Can you work these out from the model? Positions are in its coordinate system, mm. Face numbers are marked on the shaded views. A direction names the side the tool comes from. Give positions to 0.01 mm unless a question says otherwise; leave off trailing zeros. Loops run counter-clockwise (first coordinate to the right, second up) from the corner with the lowest first, then second, coordinate; pieces in that order, holes last. Notation, with made-up numbers: (2, 60.5) - (25, 60.5) arc R18 cw to (25, 84.5) - close; hole circle Ø9 at (17.5, -33.5). An arc over 180 degrees is marked (long way). Use a Markdown table: item, result. Add a question column.
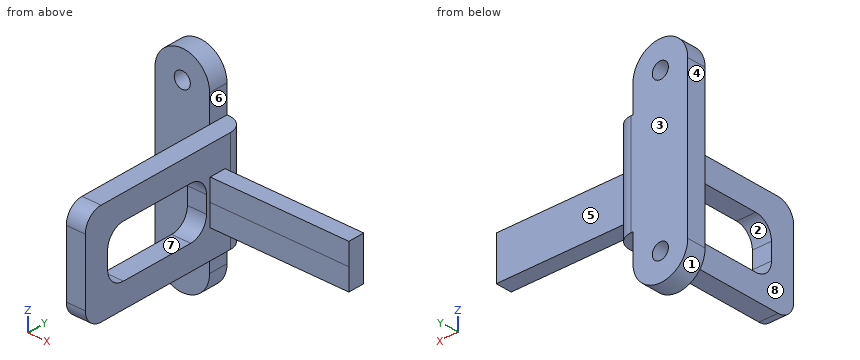
Autodesk Inventor part; units mm, degrees
ref_plane "YZ Plane" through (0, 0, 0) normal (1, 0, 0) x (0, 1, 0)
ref_plane "XZ Plane" through (0, 0, 0) normal (0, 1, 0) x (-1, 0, 0)
ref_plane "XY Plane" through (0, 0, 0) normal (0, 0, 1) x (1, 0, 0)
sketch "Sketch1" plane through (0, 0, 0) normal (0, 1, 0) x (-1, 0, 0)
  circle A0 centre (0, 0) radius 1.4732
  circle A1 centre (0, -28.4988) radius 1.4732
  circle A2 centre (0, 0) radius 5.0165
  circle A3 centre (0, -28.4988) radius 5.0165
  line L0 (5.0165, 0) -> (5.0165, -28.4988)
  line L1 (-5.0165, 0) -> (-5.0165, -28.4988)
  dimension "d0" = 2.9464
  dimension "d2" = 2.9464
  dimension "d3" = 10.033
  dimension "d4" = 10.033
extrude "Extrusion1" add sketch "Sketch1" along normal blind 3.5
sketch "Sketch2" plane through (5.0165, 0, 0) normal (1, 0, 0) x (0, 0, -1)
  line L0 (0, 0) -> (28.4988, 0)
  line L1 (0, 0) -> (5.0292, 0)
  line L2 (28.4988, 0) -> (28.4988, 3.5)
  line L3 (28.4988, 0) -> (23.4696, 0)
  line L4 (23.4696, 0) -> (5.0292, 0)
  line L5 (5.0292, 0) -> (5.0292, -25.7302)
  line L6 (8.2042, -28.9052) -> (20.2946, -28.9052)
  line L7 (23.4696, -25.7302) -> (23.4696, 0)
  line L8 (5.0292, 0) -> (23.4696, 0)
  line L9 (5.0292, 0) -> (11.3792, 0)
  line L10 (23.4696, 0) -> (17.1196, 0)
  line L11 (5.0292, -28.9052) -> (11.3792, -28.9052)
  arc A0 (5.0292, -25.7302) -> (8.2042, -28.9052) centre (8.2042, -25.7302) ccw
  arc A1 (20.2946, -28.9052) -> (23.4696, -25.7302) centre (20.2946, -25.7302) ccw
  line L12 (15.8041, -24.4147) -> (12.694, -24.4147)
  line L13 (12.694, -4.4898) -> (15.8041, -4.4898)
  line L14 (18.9791, -7.6648) -> (18.9791, -21.2397)
  line L15 (9.519, -21.2397) -> (9.519, -7.6648)
  arc A2 (12.694, -4.4898) -> (9.519, -7.6648) centre (12.694, -7.6648) ccw
  arc A3 (9.519, -21.2397) -> (12.694, -24.4147) centre (12.694, -21.2397) ccw
  arc A4 (15.8041, -24.4147) -> (18.9791, -21.2397) centre (15.8041, -21.2397) ccw
  arc A5 (18.9791, -7.6648) -> (15.8041, -4.4898) centre (15.8041, -7.6648) ccw
  point P0 (9.519, -24.4147)
  dimension "d7" = 5.0292
  dimension "d8" = 5.0292
  dimension "d9" = 28.9052
  dimension "d10" = 6.35
  dimension "d14" = 6.35
  dimension "d17" = 3.175
  dimension "d23" = 6.35
  dimension "d25" = 3.175
extrude "Extrusion4" add sketch "Sketch2" along normal blind 3.5
sketch "Sketch4" plane through (5.0165, 0, -5.0292) normal (0, 1, 0) x (1, 0, 0)
  line L0 (0, 0) -> (3.5, 0)
  line L1 (3.5, 15.2654) -> (3.5, 18.4404)
  line L2 (3.5, 0) -> (3.5, 18.4404)
  line L3 (0, 18.4404) -> (3.5, 18.4404)
  line L4 (3.5, 18.4404) -> (0, 18.4404)
  line L5 (0, 18.4404) -> (0, 0)
  line L6 (0, 0) -> (3.5, 0)
  point P0 (-5.0165, -5.0292)
extrude "Extrusion5" add sketch "Sketch4" along normal blind 3.5
fillet "Fillet3" radius 3.175 1 edges at (8.5165, 3.5, -14.2494)
sketch "Sketch5" plane through (8.5165, 0, 0) normal (1, 0, 0) x (0, 0, -1)
  line L0 (5.0292, 0) -> (23.4696, 0)
  line L1 (12.694, -4.4898) -> (15.8041, -4.4898)
  line L2 (14.2491, -3.7449) -> (10.2491, -3.7446)
  line L3 (14.2491, -3.7449) -> (18.2491, -3.7449)
  line L4 (14.2493, -0.7449) -> (10.2491, -0.7449)
  line L5 (10.2491, -0.7449) -> (10.2491, -3.7446)
  line L6 (14.2493, -0.7449) -> (18.2491, -0.7449)
  line L7 (18.2491, -0.7449) -> (18.2491, -3.7449)
  point P0 (0, 0)
extrude "Extrusion6" add sketch "Sketch5" along normal blind 25.4
properties part number "frontbackmountpi_3DPrint"
1. Suppose I cut it at A-A (x = 0). List the corners of the cut face in (y, z) for me, and give its area (3 significant figures).
2. Suppose I cut it at C-C (x = 7). List the corners of the cut face in (y, z) for me (3 decimals).
3. Please list where these lines run through material, in increasing order: line 1 along Z through (x, y) = (0, 1); line 2 along Z through (x, y) = (8, -18); line 3 along Y through (x, z) = (3.5, -4.5). Write a range as [from, to].
4. If we mould it in two halves opening along Y, with no side actions, what happens to the marked faces 1, 2 and 3? For each: released by +Y, released by -Y, zero draft, split by the parting line, or undercut.
5. Will these pins go through, and if not, where does the flat tip stop? P1, Ø6, axis at x = 14, y = -0.5, coming from the -Z side; P2, Ø2.5, axis at x = 25.5, z = -12.5, coming from the +Y side; P3, Ø1.8, axis at y = 1, z = -2, coming from the +X side; P4, Ø2.5, axis at x = 0, z = 0, coming from the -Y side.
6. On a 3-axis mill with a long thin cutter (end or side, diameter ignored), from which of +Z, -Z, +X, -X, +Y, -Y can I reach the whole of each face in a straight line? I mean the marked faces 4, 5, 6, 7 and 8. Say none if no direction works.
7. Suppose I cut it at B-B (y = -10). List the corners of the cut face in (x, z) for me.
Results below:
| question | item | result |
|---|---|---|
| 1 | outline | (0, -33.52) - (3.5, -33.52) - (3.5, -29.97) - (0, -29.97) - close; (0, -27.03) - (3.5, -27.03) - (3.5, -1.47) - (0, -1.47) - close; (0, 1.47) - (3.5, 1.47) - (3.5, 5.02) - (0, 5.02) - close |
| 1 | area | 114 mm² |
| 2 | outline | (-28.905, -20.295) arc R3.175 ccw to (-25.73, -23.47) - (3.032, -23.47) - (3.032, -5.029) - (-25.73, -5.029) arc R3.175 ccw to (-28.905, -8.204) - close; hole (-24.415, -15.804) arc R3.175 ccw to (-21.24, -18.979) - (-7.665, -18.979) arc R3.175 ccw to (-4.49, -15.804) - (-4.49, -12.694) arc R3.175 ccw to (-7.665, -9.519) - (-21.24, -9.519) arc R3.175 ccw to (-24.415, -12.694) - close |
| 3 | line 1 | [-33.52, -29.97], [-27.03, -1.47], [1.47, 5.02] |
| 3 | line 2 | [-23.47, -18.98], [-9.52, -5.03] |
| 3 | line 3 | [0, 3.5] |
| 4 | face 1 | zero draft |
| 4 | face 2 | undercut |
| 4 | face 3 | released by +Y |
| 5 | P1 | z = -18.25 |
| 5 | P2 | y = -0.74 |
| 5 | P3 | x = 5.02 |
| 5 | P4 | through |
| 6 | face 4 | +Z, -Z, -X, +Y, -Y |
| 6 | face 5 | +Z, -Z, +X, +Y |
| 6 | face 6 | +Z, +X, +Y, -Y |
| 6 | face 7 | +X, -X |
| 6 | face 8 | +Z, -Z, -X, -Y |
| 7 | outline | (5.02, -23.47) - (8.52, -23.47) - (8.52, -18.98) - (5.02, -18.98) - close; (5.02, -9.52) - (8.52, -9.52) - (8.52, -5.03) - (5.02, -5.03) - close |
